from build123d import *


with BuildPart() as part:
    # Sketch1 → Revolve1 (revolve)
    with BuildSketch(Plane.XY):
        Polygon((0, 0), (0, 8), (-40.5, 8), (-40.5, 6), (-65, 6), (-65, 0), align=None)
    revolve1 = revolve(axis=Axis((-65, 0, 0), (1, 0, 0)))

    # Mirror1: Revolve1 across plane
    add(revolve1.mirror(Plane.ZY))


solid = part.part
Design review of the part built by this model. Coordinates are the model's own, in mm. A direction names the side the tool comes from. Round coordinates to 2 decimals unless told otherwise and drop trailing zeros. Write each loop counter-clockwise with the first axis right and the second up, starting at its lowest first coordinate (ties: lowest second). Pieces come first, ordered by that corner, then holes.
Item 1: Wall thickness on L1, parallel to Z at x = 47.5, y = -0.5; L2, parallel to Y at x = -17.5, z = -0.5; L3, parallel to X at y = 5, z = -3.5: over which ranges is each line inside the solid? List them lowest first.
Item 2: For faces 1 (the cylindrical face through (-53, -6, 0)), 2 (the flat face through (40.5, -2, 6)), 3 (the flat face through (65, 0, 0)), list the 3-axis set-ups (+Z, -Z, +X, -X, +Y, -Y) from which the entire face can be reached by the end or side of a thin tool; tool diameter is ignored.
Item 3: Consider section C-C on x = -3.5. Give the boundary of the cut face in (y, z).
Item 4: For pin 1 Ø8 at (x, z) = (45.5, 3.5) entering from -Y; pin 2 Ø5 at (x, y) = (-44.5, 6) entering from -Z, all flat-tipped, find the tip position at first contact; note any pin that passes through.
Item 5: Consider section D-D on x = 55. Give the boundary of the cut face in (y, z).
Item 6: Consider section A-A on y = 0. Give the boundary of the cut face in (x, z), and give its area (3 significant figures).
Check values:
1. L1: z = -5.98 to 5.98
1. L2: y = -7.98 to 7.98
1. L3: x = -40.5 to 40.5
2. face 1: -X
2. face 2: +X
2. face 3: +Z, -Z, +X, +Y, -Y
3. outline: circle Ø16 at (0, 0)
4. pin 1: stops at y = -6
4. pin 2: stops at z = -4.87
5. outline: circle Ø12 at (0, 0)
6. outline: (-65, -6) - (-40.5, -6) - (-40.5, -8) - (40.5, -8) - (40.5, -6) - (65, -6) - (65, 6) - (40.5, 6) - (40.5, 8) - (-40.5, 8) - (-40.5, 6) - (-65, 6) - close
6. area: 1,880 mm2
